from build123d import *

# Parameters (mm, degrees)
SKETCH1_R                = 9.55
TUBEINTERFACE1_DEPTH     = 5
SKETCH3_R                = 10.8
BODY_DEPTH               = 7
BODYCHAMFER_SIZE         = 0.2
SKETCH4_W                = 10
SKETCH4_H                = 75
FLATS_DEPTH              = 3
SKETCH27_R               = 7
HEADCOVERBORE_DEPTH      = 3
SKETCH28_R               = 4.639
INLINE_PORT_DEPTH        = 20.423696867
INLINE_PORT_CHAMFER_SIZE = 0.5
CHAMFER4_SIZE            = 0.5
CHAMFER4_SIZE2           = 0.866025404


with BuildPart() as part:
    # Sketch1 → TubeInterface1 (new body)
    with BuildSketch(Plane.XY):
        Circle(SKETCH1_R)
    extrude(amount=TUBEINTERFACE1_DEPTH)

    # Sketch3 → Body (add)
    with BuildSketch(Plane.XY.offset(5)):
        Circle(SKETCH3_R)
    extrude(amount=BODY_DEPTH)

    # BodyChamfer
    bodychamfer_edges = [part.edges().sort_by_distance(p)[0] for p in [
        (-10.8, 0, 12),
    ]]
    chamfer(bodychamfer_edges, length=BODYCHAMFER_SIZE)

    # Sketch4 → Flats (cut)
    with BuildSketch(Plane.XY.offset(12)):
        with Locations((-12.9, 0)):
            Rectangle(SKETCH4_W, SKETCH4_H)
        with Locations((12.9, 0)):
            Rectangle(SKETCH4_W, SKETCH4_H)
    extrude(amount=-FLATS_DEPTH, mode=Mode.SUBTRACT)

    # Sketch23 → RodCoverCrimp (revolve, cut)
    with BuildSketch(Plane(origin=(0, 0, 0), x_dir=(0, 0, -1), z_dir=(1, 0, 0)), mode=Mode.PRIVATE) as rodcovercrimp_sk:
        Polygon((-7.5, 13.6), (-5, 13.6), (-5, 10.2), (-5.5, 10.2), (-7.1, 8.6), (-7.5, 8.6), align=None)
    revolve(rodcovercrimp_sk.sketch.rotate(Axis((0, 0, 0), (0, 0, -1)), 90), axis=Axis((0, 0, 0), (0, 0, -1)), mode=Mode.SUBTRACT)

    # Sketch24 → TubeInterfaceCrimp (revolve, cut)
    with BuildSketch(Plane(origin=(0, 0, 0), x_dir=(0, 0, -1), z_dir=(1, 0, 0)), mode=Mode.PRIVATE) as tubeinterfacecrimp_sk:
        Polygon((-5, 34.292463075), (-5, 8.6), (-4.1, 8.6), (-3.15, 9.55), (0, 9.55), (0, 34.292463075), align=None)
    revolve(tubeinterfacecrimp_sk.sketch.rotate(Axis((0, 0, 0), (0, 0, -1)), 90), axis=Axis((0, 0, 0), (0, 0, -1)), mode=Mode.SUBTRACT)

    # Sketch27 → HeadCoverBore (cut)
    with BuildSketch(Plane(origin=(0, 0, 0), x_dir=(-1, 0, 0), z_dir=(0, 0, -1))):
        Circle(SKETCH27_R)
    extrude(amount=-HEADCOVERBORE_DEPTH, mode=Mode.SUBTRACT)

    # Sketch28 → Inline Port (cut, through all)
    with BuildSketch(Plane.XY.offset(12)):
        Circle(SKETCH28_R)
    extrude(amount=-INLINE_PORT_DEPTH, mode=Mode.SUBTRACT)

    # Inline Port Chamfer
    inline_port_chamfer_edges = [part.edges().sort_by_distance(p)[0] for p in [
        (-4.639, 0, 12),
    ]]
    chamfer(inline_port_chamfer_edges, length=INLINE_PORT_CHAMFER_SIZE)

    # Chamfer4
    chamfer4_edges = [part.edges().sort_by_distance(p)[0] for p in [
        (-9.55, 0, 0),
    ]]
    chamfer4_side = [part.faces().sort_by_distance(p)[0] for p in [
        (-9.27988521, 0, 0),
    ]]
    chamfer(chamfer4_edges, length=CHAMFER4_SIZE, length2=CHAMFER4_SIZE2, reference=chamfer4_side[0])


solid = part.part
Model file for the job. Use its own axes, mm. A direction names the side the tool comes from. Round coordinates to 2 decimals unless told otherwise and drop trailing zeros. Loops run counter-clockwise (first coordinate to the right, second up) from the corner with the lowest first, then second, coordinate; pieces in that order, holes last.
1. Band-saw the part on B-B, the plane z = 4.5. List the corners of the cut face in (x, y), and give its area (3 significant figures).
Check values:
outline: circle Ø17.2 at (0, 0); hole circle Ø9.28 at (0, 0)
area: 165 mm2
2. Tool access for faces 1 (the cylindrical face through (-0.6, 4.6, 7.3)), 2 (the cylindrical face through (9.73, -3.06, 5.25)), 3 (the flat face through (-9, 0, 9)), 4 (the flat face through (-5, -8, 5)): list every direction of +Z, -Z, +X, -X, +Y, -Y with a clear straight run to the whole face (end or side of a thin tool).
Check values:
face 1: +Z, -Z
face 2: -Z
face 3: +Z, -X, +Y, -Y
face 4: none
3. Mould opens along Z. For faces 5 (the flat face through (7.9, 0, 11)), 6 (the flat face through (9, 0, 9)), 7 (the flat face through (1, 9, 7.5)) say: +Z half, -Z half, draft (parallel to the pull), parting line (faces both ways), or undercut.
Check values:
face 5: draft
face 6: +Z half
face 7: undercut
4. Band-saw the part on D-D, the plane z = 2. List the corners of the cut face in (x, y), and give its area (3 significant figures).
Check values:
outline: circle Ø19.1 at (0, 0); hole circle Ø14 at (0, 0)
area: 133 mm2
5. Drop flat-ended pins along their axis: P1, Ø12.5, axis at x = 0, y = 0, coming from the -Z side; P2, Ø1.5, axis at x = 4.5, z = 4.5, coming from the +Y side; P3, Ø2.5, axis at y = 1.5, z = 10.5, coming from the +X side; P4, Ø8.5, axis at x = 0, y = 0, coming from the -Z side. Give the stop position or say it passes through.
Check values:
P1: stops at z = 3
P2: stops at y = 9.41
P3: stops at x = 7.9
P4: passes through
6. Wall check: probe 1 along Y at (x, z) = (0, 2.4); probe 2 along Y at (x, z) = (0, 5.25); probe 3 along Z at (x, y) = (-1, 9.25). Give the ranges that are in metal, low to high.
Check values:
probe 1: y = -9.55 to -7, 7 to 9.55
probe 2: y = -10.2 to -4.64, 4.64 to 10.2
probe 3: z = 0.44 to 3.4, 5 to 6.4, 7.5 to 12
7. Band-saw the part on C-C, the plane z = 10. List the corners of the cut face in (x, y).
Check values:
outline: (-7.9, -7.36) arc R10.8 ccw to (7.9, -7.36) - (7.9, 7.36) arc R10.8 ccw to (-7.9, 7.36) - close; hole circle Ø9.28 at (0, 0)
